Job drawing, mm, ordinate dimensions from the low corner. One solid piece. A direction names the side the tool comes from. Round coordinates to 2 decimals unless told otherwise and drop trailing zeros. Write each loop counter-clockwise with the first axis right and the second up, starting at its lowest first coordinate (ties: lowest second). Pieces come first, ordered by that corner, then holes.
1) Which spindle directions (+Z, -Z, +X, -X, +Y, -Y) get a long thin tool onto all of the face, cutting with end or side? Do the marked faces 4, 5 and 6. Say none if no direction does.
2) Saw through at C-C on z = 66. Write the cut outline in (x, y), and give its area (3 significant figures).
3) Saw through at B-B on y = 33. Write the cut outline in (x, z), and give its area (3 significant figures).
4) Drill centre lines: L1, parallel to Z at x = 35, y = 30.5; L2, parallel to Y at x = 55, z = 142.5 (3 decimals); L3, parallel to Y at x = 92, z = 75.5. Where is each one in solid material? Low to high.
5) Pull direction Z, two halves, no side cores. Call the marked faces 1, 2 and 3: +Z half, -Z half, draft (parallel to the pull), parting line (faces both ways), or undercut.
6) Saw through at A-A on x = 53.5. Write the cut outline in (y, z).
7) Saw through at D-D on y = 69. Write the cut outline in (x, z), and give its area (3 significant figures).
8) Flat gauge pins, fed straight in: pin 1 (8 mm diameter, centred on x = 85.5, y = 56, fed in from +Z); pin 2 (12 mm diameter, centred on y = 67.5, z = 75, fed in from +X); pin 3 (8 mm diameter, centred on x = 21, y = 17.5, fed in from -Z). Where does each tip first touch, or does it go through?
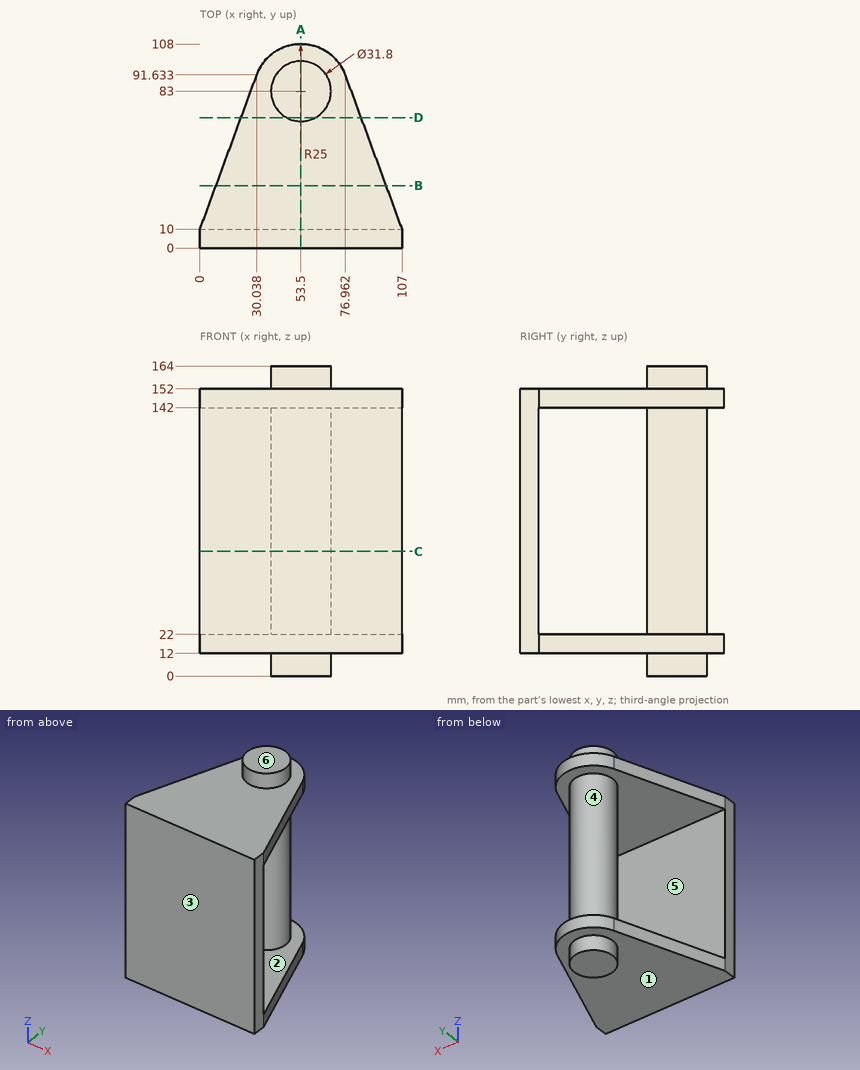
Completed:
1. face 4: none
1. face 5: +X, -X
1. face 6: +Z, +X, -X, +Y, -Y
2. outline: (0, 0) - (107, 0) - (107, 10) - (0, 10) - close; circle Ø31.8 at (53.5, 83)
2. area: 1,860 mm2
3. outline: (8.46, 12) - (98.54, 12) - (98.54, 22) - (8.46, 22) - close; (8.46, 142) - (98.54, 142) - (98.54, 152) - (8.46, 152) - close
3. area: 1,800 mm2
4. L1: z = 12 to 22, 142 to 152
4. L2: y = 0 to 107.955
4. L3: y = 0 to 10
5. face 1: -Z half
5. face 2: undercut
5. face 3: draft
6. outline: (0, 12) - (67.1, 12) - (67.1, 0) - (98.9, 0) - (98.9, 12) - (108, 12) - (108, 22) - (98.9, 22) - (98.9, 142) - (108, 142) - (108, 152) - (98.9, 152) - (98.9, 164) - (67.1, 164) - (67.1, 152) - (0, 152) - close; hole (10, 22) - (67.1, 22) - (67.1, 142) - (10, 142) - close
7. outline: (21.71, 12) - (45.96, 12) - (45.96, 0) - (61.04, 0) - (61.04, 12) - (85.29, 12) - (85.29, 22) - (61.04, 22) - (61.04, 142) - (85.29, 142) - (85.29, 152) - (61.04, 152) - (61.04, 164) - (45.96, 164) - (45.96, 152) - (21.71, 152) - (21.71, 142) - (45.96, 142) - (45.96, 22) - (21.71, 22) - close
7. area: 3,440 mm2
8. pin 1: stops at z = 152
8. pin 2: stops at x = 66.25
8. pin 3: stops at z = 12
